Answer from the drawing. Dimensions are ordinates in mm from the lowest x, y and z of the part. A direction names the side the tool comes from. Coordinates: 2 decimals unless noted, no trailing zeros. Order: outer loops, then holes, each group sorted by start corner. A loop starts at its lowest first (then second) coordinate and runs counter-clockwise, first axis right, second up. Notation, with made-up numbers: (-11, 45) - (-4, 45) arc R14 ccw to (-4, 49) - close; hole circle Ø4 at (87, 62). An arc over 180 degrees is marked (long way). Answer as a JSON object with one key per item and string values. Group by question number.
1) The mould has two halves that part along Z. Classify the marked faces 1, 2, 3 and 4: released by +Z, released by -Z, zero draft, split by the parting line, or undercut.
2) Section C-C (x = 5) is taken. Give the vertices of the cut face in (y, z).
3) Section A-A (x = 105) is taken. Give the vertices of the cut face in (y, z), plus the area to 3 significant figures.
4) A tool of negligible diameter and unlimited length cuts with its end or side. For the marked faces 5, 6, 7, 8 and 9, from which of +Z, -Z, +X, -X, +Y, -Y can it reach the whole face along a straight path? Write none if from no direction.
5) Section D-D (z = 26.5) is taken. Give the vertices of the cut face in (x, y).
6) Section B-B (y = 1) is taken. Give the vertices of the cut face in (x, z).
7) Find the intervals of material crossed by line 1 along Y through (x, z) = (105, 34.85); line 2 along X through (y, z) = (4, 35.5); line 3 along X through (y, z) = (4.75, 35) (1 decimal), in increasing order.
8) Each of these flat-tipped pins is pushed along its axis until it touches: P1, Ø5, axis at y = 6.5, z = 15, coming from the +X side; P2, Ø2, axis at x = 56.5, y = 2, coming from the +Z side; P3, Ø4.5, axis at x = 28.5, y = 3.5, coming from the -Z side (1 decimal). Where does it stop, or does it pass through?
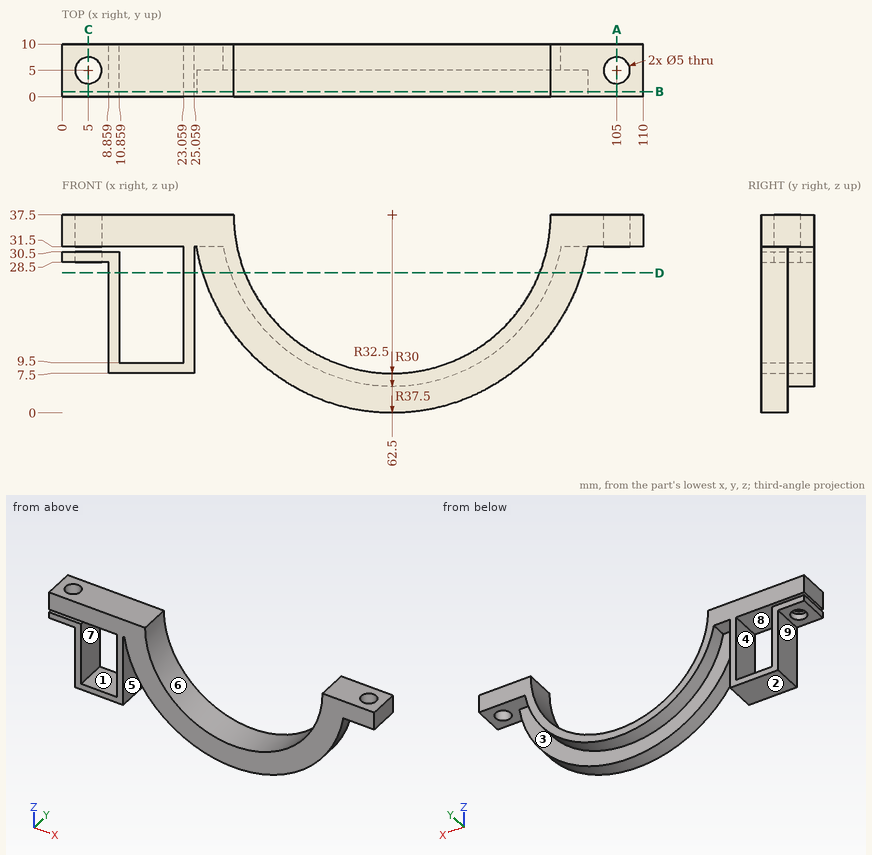
Report:
{
 "1": {"face 1": "undercut", "face 2": "released by -Z", "face 3": "zero draft", "face 4": "undercut"},
 "2": {"outline": "(0, 28.5) - (2.5, 28.5) - (2.5, 30.5) - (0, 30.5) - close; (0, 31.5) - (2.5, 31.5) - (2.5, 37.5) - (0, 37.5) - close; (7.5, 28.5) - (10, 28.5) - (10, 30.5) - (7.5, 30.5) - close; (7.5, 31.5) - (10, 31.5) - (10, 37.5) - (7.5, 37.5) - close"},
 "3": {"outline": "(0, 31.5) - (2.5, 31.5) - (2.5, 37.5) - (0, 37.5) - close; (7.5, 31.5) - (10, 31.5) - (10, 37.5) - (7.5, 37.5) - close", "area": "30.0 mm²"},
 "4": {"face 5": "-Z, +Y, -Y", "face 6": "+Z, +Y, -Y", "face 7": "+Y, -Y", "face 8": "-X, +Y, -Y", "face 9": "-Z, -X, +Y, -Y"},
 "5": {"outline": "(8.86, 0) - (10.86, 0) - (10.86, 10) - (8.86, 10) - close; (23.06, 0) - (25.06, 0) - (25.06, 10) - (23.06, 10) - close; (26.65, 0) - (34.59, 0) - (34.59, 10) - (31.92, 10) - (31.92, 5) - (26.65, 5) - close; (90.41, 0) - (98.35, 0) - (98.35, 5) - (93.08, 5) - (93.08, 10) - (90.41, 10) - close"},
 "6": {"outline": "(0, 28.5) - (8.86, 28.5) - (8.86, 7.5) - (25.06, 7.5) - (25.06, 31.5) - (25.48, 31.5) arc R37.5 ccw to (99.52, 31.5) - (110, 31.5) - (110, 37.5) - (92.5, 37.5) arc R30 cw to (32.5, 37.5) - (0, 37.5) - (0, 31.5) - (23.06, 31.5) - (23.06, 9.5) - (10.86, 9.5) - (10.86, 30.5) - (0, 30.5) - close"},
 "7": {"line 1": "y = 0 to 2.5, 7.5 to 10", "line 2": "x = 0 to 2.71, 7.29 to 32.57, 92.43 to 102.71, 107.29 to 110", "line 3": "x = 0 to 2.5, 7.5 to 32.6, 92.4 to 102.5, 107.5 to 110"},
 "8": {"P1": "stops at x = 93.9", "P2": "stops at z = 8.33", "P3": "stops at z = 17.5"}
}
